from build123d import *

# Parameters (mm, degrees)
F1_DEPTH = 76.2
F2_R     = 10


with BuildPart() as f1:
    # F0 (on Top) → F1 (new body)
    with BuildSketch(Plane.XY):
        Polygon((75.046457, 811.90747), (0, 812.8), (0, 0), (79.210013, 0), (79.210013, -68.688758), (162.481502, -68.688758), (162.481502, 0), (228.6, 0), (228.6, 812.8), (158.317953, 811.90747), (158.317953, 886.851847), (75.046457, 886.851847), align=None)
    extrude(amount=F1_DEPTH)

    # F2
    f2_edges = [f1.edges().sort_by_distance(p)[0] for p in [
        (75.046457, 886.851847, 38.1),
        (116.682205, 886.851847, 76.2),
        (75.046457, 849.379659, 76.2),
        (158.317953, 849.379659, 76.2),
        (158.317953, 886.851847, 38.1),
        (116.682205, 886.851847, 0),
        (75.046457, 849.379659, 0),
        (158.317953, 849.379659, 0),
    ]]
    fillet(f2_edges, radius=F2_R)


solid = f1.part
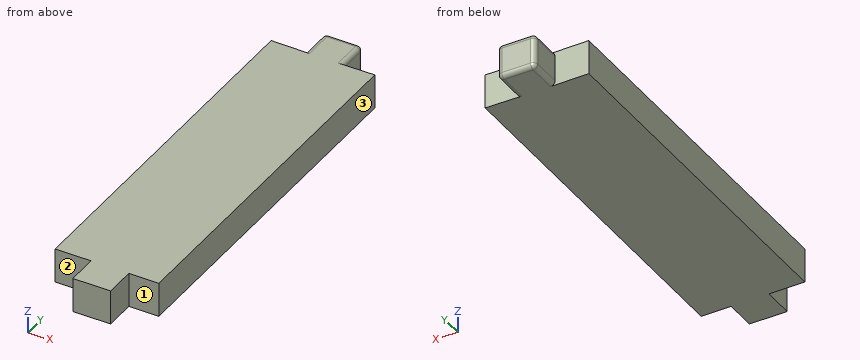
Read the model definition and answer for the solid it produces. Units are mm, in the model's axes. Face numbers are marked on the shaded views. A direction names the side the tool comes from. Give positions to 0.01 mm unless a question says otherwise; leave off trailing zeros. Loops run counter-clockwise (first coordinate to the right, second up) from the corner with the lowest first, then second, coordinate; pieces in that order, holes last. Notation, with made-up numbers: M 55,18.5 L 113,18.5 A16 ccw 113,47.5 Z; hole C 77.5,-39.5 d2. An arc over 180 degrees is marked long. Write each question's results on one line, items separated by ' | '.
1. Section A-A on z = 50 is taken. Give the vertices of the cut face in (x, y).
Values:
outline: M 0,0 L 79.21,0 L 79.21,-68.69 L 162.48,-68.69 L 162.48,0 L 228.6,0 L 228.6,812.8 L 158.32,811.91 L 158.32,876.85 A10 ccw 148.32,886.85 L 85.05,886.85 A10 ccw 75.05,876.85 L 75.05,811.91 L 0,812.8 Z
2. Straight lines are drawn through the part: line 1 (Y direction, x = 164.5, z = 33); line 2 (Y direction, x = 160, z = 40). For each, find the intervals that lie inside material, in ascending order. Write a range as [from, to].
Values:
line 1: y = [0, 811.99] | line 2: y = [-68.69, 811.93]
3. A tool of negligible diameter and unlimited length cuts with its end or side. For the marked faces 1, 2 and 3, from which of +Z, -Z, +X, -X, +Y, -Y can it reach the whole face along a straight path? Write none if from no direction.
Values:
face 1: +Z, -Z, +X, -Y | face 2: +Z, -Z, -X, -Y | face 3: +Z, -Z, +X, +Y, -Y
4. Section B-B on x = 176.5 is taken. Give the vertices of the cut face in (y, z), plus the area to 3 significant figures.
Values:
outline: M 0,0 L 812.14,0 L 812.14,76.2 L 0,76.2 Z | area: 61,900 mm^2
5. Section C-C on x = 58 is taken. Give the vertices of the cut face in (y, z).
Values:
outline: M 0,0 L 812.11,0 L 812.11,76.2 L 0,76.2 Z
